The listing builds one solid part. Answer for the finished solid, in the listing's coordinates (mm). A direction names the side the tool comes from. Give positions to 0.01 mm unless a question says otherwise; leave off trailing zeros. Loops run counter-clockwise (first coordinate to the right, second up) from the corner with the lowest first, then second, coordinate; pieces in that order, holes last. Notation, with made-up numbers: M 28,9.25 L 87,9.25 A31 ccw 87,40.25 Z; hole C -3.5,-7.75 d10. An arc over 180 degrees is marked long. One line per item, written item: value. Start each with the question number.
Q1. Flat-ended cylindrical pins translate along their axes: pin 1 (7 mm diameter, centred on x = -59, y = 56.5, fed in from +Z); pin 2 (4 mm diameter, centred on y = 57.5, z = 26, fed in from +X); pin 3 (1 mm diameter, centred on x = -1.5, y = 47.5, fed in from -Z). Find the tip coordinate at first contact, or state that the pin passes through.
Q2. The mould has two halves that part along Z. Classify faces 4 (the flat face through (68, 38, 45)), 5 (the flat face through (-54, 38, 50)), 6 (the cylindrical face through (-49.104, 38.454, -9.421)), 7 (the flat face through (-39.6, 38.454, -41.014)): +Z half, -Z half, draft (parallel to the pull), parting line (faces both ways), or undercut.
Q3. A cutting plane is placed at C-C, the plane x = 0. Determine the outline of the cut face in (y, z), and give its area (3 significant figures).
Q4. A cutting plane is placed at B-B, the plane x = 59. Determine the outline of the cut face in (y, z).
Q5. For faces 1 (the flat face through (59, 38, 40)), 2 (the flat face through (-59, 38, 40)), 3 (the cylindrical face through (-61.08, 52.51, 44.93)), determine the directions among +Z, -Z, +X, -X, +Y, -Y from which every point of the face is accessible in a straight line to the end or side of a thin tool.
Q6. A cutting plane is placed at A-A, the plane y = 56.5. Determine the outline of the cut face in (x, z).
Q7. Consider L1, parallel to Y at x = -59, z = 47.25; L2, parallel to Y at x = 59, z = 45.5; L3, parallel to Z at x = -37, y = 10.5. Determine where each line is inside the solid, lowest interval first.
Q8. A cutting plane is placed at D-D, the plane z = -10. Determine the outline of the cut face in (x, y), and give its area (3 significant figures).
from build123d import *

# Parameters (mm, degrees)
BOSS_EXTRUDE2_DEPTH      = 78
M8_CLEARANCE_HOLE1_D     = 9
M8_CLEARANCE_HOLE1_DEPTH = 10
M8_CLEARANCE_HOLE1_TIP   = 2.703872786
M8_CLEARANCE_HOLE2_D     = 9


with BuildPart() as part:
    # Sketch1 → Boss-Extrude2 (new body)
    with BuildSketch(Plane(origin=(0, 0, 0), x_dir=(1, 0, 0), z_dir=(0, 1, 0))):
        with BuildLine():
            Line((-68, -50), (-50, -50))
            Line((-50, -50), (-40, -50))
            Line((-40, -50), (-30, -40))
            ThreePointArc((-30, -40), (0, -50), (30, -40))
            Line((30, -40), (40, -50))
            Line((40, -50), (50, -50))
            Line((50, -50), (68, -50))
            Line((68, -50), (68, -40))
            Line((68, -40), (50, -40))
            Line((50, -40), (50, 0))
            ThreePointArc((50, 0), (28.168436295, 41.310279553), (-18.261567868, 46.545839116))
            Line((-18.261567868, 46.545839116), (-37.864743155, 66.149014403))
            Line((-37.864743155, 66.149014403), (-51.299771998, 52.71398556))
            Line((-51.299771998, 52.71398556), (-27.56832425, 28.982537812))
            ThreePointArc((-27.56832425, 28.982537812), (15.76811704, 36.760936944), (40, 0))
            ThreePointArc((40, 0), (-14.84416531, -37.143650282), (-28.982537812, 27.56832425))
            Line((-28.982537812, 27.56832425), (-52.71398556, 51.299771998))
            Line((-52.71398556, 51.299771998), (-66.149014403, 37.864743155))
            Line((-66.149014403, 37.864743155), (-46.545839116, 18.261567868))
            ThreePointArc((-46.545839116, 18.261567868), (-49.128871124, 9.292686485), (-50, 0))
            Line((-50, 0), (-50, -40))
            Line((-50, -40), (-68, -40))
            Line((-68, -40), (-68, -50))
        make_face()
    extrude(amount=BOSS_EXTRUDE2_DEPTH)

    # M8 Clearance Hole1
    with Locations(Plane.XY.offset(50)):
        with Locations((-59, 69.5), (-59, 7), (-59, 56.5), (59, 56.5), (59, 8.5), (59, 69.5)):
            Hole(M8_CLEARANCE_HOLE1_D / 2, depth=M8_CLEARANCE_HOLE1_DEPTH)
            with Locations((0, 0, -(M8_CLEARANCE_HOLE1_DEPTH + M8_CLEARANCE_HOLE1_TIP / 2))):  # 118° drill point
                Cone(0, M8_CLEARANCE_HOLE1_D / 2, M8_CLEARANCE_HOLE1_TIP, mode=Mode.SUBTRACT)

    # M8 Clearance Hole2 (through all)
    with Locations(Plane(origin=(14.142135624, 0, -14.142135624), x_dir=(-0.707106781, 0, -0.707106781), z_dir=(0.707106781, 0, -0.707106781))):
        with Locations((59.687295128, 8.5), (59.687295128, 69.5)):
            Hole(M8_CLEARANCE_HOLE2_D / 2)


solid = part.part
Answer block:
1. pin 1: z = -27.22
1. pin 2: x = 50
1. pin 3: z = -49.99
2. face 4: draft
2. face 5: +Z half
2. face 6: undercut
2. face 7: undercut
3. outline: M 0,-50 L 78,-50 L 78,-40 L 0,-40 Z; M 0,40 L 78,40 L 78,50 L 0,50 Z
3. area: 1,560 mm^2
4. outline: M 0,40 L 4,40 L 4,50 L 0,50 Z; M 13,40 L 52,40 L 52,50 L 13,50 Z; M 61,40 L 65,40 L 65,50 L 61,50 Z; M 74,40 L 78,40 L 78,50 L 74,50 Z
5. face 1: -Z, +X, +Y, -Y
5. face 2: -X, +Y, -Y
5. face 3: +Z
6. outline: M -68,40 L -63.5,40 L -63.5,50 L -68,50 Z; M -66.15,-37.86 L -52.71,-51.3 L -28.98,-27.57 A40 cw long -27.57,-28.98 L -51.3,-52.71 L -37.86,-66.15 L -18.26,-46.55 A50 ccw 50,0 L 50,40 L 54.5,40 L 54.5,50 L 40,50 L 30,40 A50 ccw -30,40 L -40,50 L -54.5,50 L -54.5,40 L -50,40 L -50,0 A50 ccw -46.55,-18.26 Z; M 63.5,40 L 68,40 L 68,50 L 63.5,50 Z
7. L1: 0 to 2.5, 11.5 to 52, 61 to 65, 74 to 78
7. L2: 0 to 4, 13 to 52, 61 to 65, 74 to 78
7. L3: -65.28 to -53.11, -41.71 to -38.41, -35.59 to -15.2, 15.2 to 47
8. outline: M -48.99,0 L -38.73,0 L -38.73,78 L -48.99,78 Z; M 38.73,0 L 48.99,0 L 48.99,78 L 38.73,78 Z
8. area: 1,600 mm^2
